from build123d import *

# Parameters (mm, degrees)
SKETCH1_W                                           = 150
SKETCH1_H                                           = 60
SKETCH1_W_2                                         = 20
SKETCH1_H_2                                         = 40
BOSS_EXTRUDE1_DEPTH                                 = 6
CBORE_FOR_M4_HEX_SOCKET_HEAD_CAP_SCREW1_D           = 4.5
CBORE_FOR_M4_HEX_SOCKET_HEAD_CAP_SCREW1_CBORE_D     = 8
CBORE_FOR_M4_HEX_SOCKET_HEAD_CAP_SCREW1_CBORE_DEPTH = 4.4
M4_CLEARANCE_HOLE1_D                                = 4.5
M4_CLEARANCE_HOLE1_DEPTH                            = 8.499


with BuildPart() as part:
    # Sketch1 → Boss-Extrude1 (new body)
    with BuildSketch(Plane(origin=(0, 0, 0), x_dir=(1, 0, 0), z_dir=(0, 1, 0))):
        Rectangle(SKETCH1_W, SKETCH1_H)
        Rectangle(SKETCH1_W_2, SKETCH1_H_2, mode=Mode.SUBTRACT)
    extrude(amount=BOSS_EXTRUDE1_DEPTH)

    # CBORE for M4 Hex Socket Head Cap Screw1 (through all)
    with Locations(Plane(origin=(0, 0, 178.229982134), x_dir=(0, 0, 1), z_dir=(0, -1, 0))):
        with Locations((-168.229982134, -69.75), (-188.229982134, -69.75)):
            cbore_for_m4_hex_socket_head_cap_screw1 = CounterBoreHole(CBORE_FOR_M4_HEX_SOCKET_HEAD_CAP_SCREW1_D / 2, CBORE_FOR_M4_HEX_SOCKET_HEAD_CAP_SCREW1_CBORE_D / 2, CBORE_FOR_M4_HEX_SOCKET_HEAD_CAP_SCREW1_CBORE_DEPTH)

    # Mirror2: CBORE for M4 Hex Socket Head Cap Screw1 across plane
    add(cbore_for_m4_hex_socket_head_cap_screw1.mirror(Plane.ZY), mode=Mode.SUBTRACT)

    # M4 Clearance Hole1
    with Locations(Plane(origin=(0, 6, 178.229982134), x_dir=(0, 0, -1), z_dir=(0, 1, 0))):
        with Locations((153.479982134, 4.75), (153.479982134, -4.75), (202.479982134, -4.75), (202.479982134, 4.75)):
            Hole(M4_CLEARANCE_HOLE1_D / 2, depth=M4_CLEARANCE_HOLE1_DEPTH)


solid = part.part
Part model, mm, in its own coordinate system. A direction names the side the tool comes from. Give positions to 0.01 mm unless a question says otherwise; leave off trailing zeros. Write each loop counter-clockwise with the first axis right and the second up, starting at its lowest first coordinate (ties: lowest second). Pieces come first, ordered by that corner, then holes.
1) Which spindle directions (+Z, -Z, +X, -X, +Y, -Y) get a long thin tool onto all of the face, cutting with end or side? Do faces 1 (the face through (-71.5, 4.4, 11.7)), 2 (the face through (-10, 3, 0)), 3 (the face through (-1, 3, -30)). Say none if no direction does.
Resolved:
face 1: -Y
face 2: +Y, -Y
face 3: -Z, +X, -X, +Y, -Y
2) Pin check, flat tip, straight feed: pin 1 (10.5 mm diameter, centred on x = -69.75, z = 10, fed in from -Y). Stop position of the tip, or through.
Resolved:
pin 1: stops at y = 0
3) Probe L1, parallel to X at y = 4.35, z = -24; L2, parallel to X at y = 2.85, z = 10; L3, parallel to Z at x = -69.75, y = 2.95. List the from-to ranges inside material, lowest first.
Resolved:
L1: x = -75 to -6.99, -2.51 to 2.51, 6.99 to 75
L2: x = -75 to -73.75, -65.75 to -10, 10 to 65.75, 73.75 to 75
L3: z = -30 to -14, -6 to 6, 14 to 30
4) Two-plate mould, pull along Z, no slides. Class faces 4 (the face through (4.074, 2.958, 26.896)), 5 (the face through (75, 3, 0)), 6 (the face through (-1, 3, 30)): released by +Z, released by -Z, zero draft, split by the parting line, or undercut.
Resolved:
face 4: undercut
face 5: zero draft
face 6: released by +Z
5) Cut at A-A on z = -24.25. Write the cut outline in (x, y), then the cut area to 3 significant figures.
Resolved:
outline: (-75, 0) - (-7, 0) - (-7, 6) - (-75, 6) - close; (-2.5, 0) - (2.5, 0) - (2.5, 6) - (-2.5, 6) - close; (7, 0) - (75, 0) - (75, 6) - (7, 6) - close
area: 846 mm2
6) Cut at D-D on x = -69.75. Write the cut outline in (y, z), then the cut area to 3 significant figures.
Resolved:
outline: (0, -30) - (6, -30) - (6, -12.25) - (4.4, -12.25) - (4.4, -14) - (0, -14) - close; (0, -6) - (4.4, -6) - (4.4, -7.75) - (6, -7.75) - (6, 7.75) - (4.4, 7.75) - (4.4, 6) - (0, 6) - close; (0, 14) - (4.4, 14) - (4.4, 12.25) - (6, 12.25) - (6, 30) - (0, 30) - close
area: 275 mm2
7) Cut at C-C on z = -10. Write the cut outline in (x, y).
Resolved:
outline: (-75, 0) - (-73.75, 0) - (-73.75, 4.4) - (-72, 4.4) - (-72, 6) - (-75, 6) - close; (-67.5, 4.4) - (-65.75, 4.4) - (-65.75, 0) - (-10, 0) - (-10, 6) - (-67.5, 6) - close; (10, 0) - (65.75, 0) - (65.75, 4.4) - (67.5, 4.4) - (67.5, 6) - (10, 6) - close; (72, 4.4) - (73.75, 4.4) - (73.75, 0) - (75, 0) - (75, 6) - (72, 6) - close
8) Cut at B-B on x = -4.75. Write the cut outline in (y, z).
Resolved:
outline: (0, -30) - (6, -30) - (6, -26.5) - (0, -26.5) - close; (0, -22) - (6, -22) - (6, -20) - (0, -20) - close; (0, 20) - (6, 20) - (6, 22.5) - (0, 22.5) - close; (0, 27) - (6, 27) - (6, 30) - (0, 30) - close
